from build123d import *

# Parameters (mm, degrees)
SKETCH_1_W          = 7
SKETCH_1_H          = 13
SKETCH_1_H_2        = 2
EXTRUDE_1_DEPTH     = 7
SKETCH_2_W          = 7
SKETCH_2_H          = 7
CUT_EXTRUDE_1_DEPTH = 3.5
FILLET_1_R          = 3.5
SKETCH_3_R          = 1.5
CUT_EXTRUDE_2_DEPTH = 13.835497653
SKETCH_4_R          = 1.5
CUT_EXTRUDE_3_DEPTH = 17.740669043
FILLET_2_R          = 2
FILLET_3_R          = 0.8


with BuildPart() as part:
    # 草图1 → 凸台-拉伸1 (new body)
    with BuildSketch(Plane.XY):
        with BuildLine():
            Line((-8.5, -6.5), (-3.5, -6.5))
            Line((-3.5, -6.5), (-3.5, -1.5))
            ThreePointArc((-3.5, -1.5), (-4.964466094, -5.035533906), (-8.5, -6.5))
        make_face()
        Rectangle(SKETCH_1_W, SKETCH_1_H)
        with Locations((7, -5.5)):
            Rectangle(SKETCH_1_W, SKETCH_1_H_2)
    extrude(amount=EXTRUDE_1_DEPTH)

    # 草图2 → 切除-拉伸1 (cut)
    with BuildSketch(Plane.XY.offset(7)):
        with Locations((0, 3)):
            Rectangle(SKETCH_2_W, SKETCH_2_H)
    extrude(amount=-CUT_EXTRUDE_1_DEPTH, mode=Mode.SUBTRACT)

    # 圆角1
    fillet_1_edges = [part.edges().sort_by_distance(p)[0] for p in [
        (10.5, -5.5, 0),
        (10.5, -5.5, 7),
        (3.5, 6.5, 1.75),
        (-3.5, 6.5, 1.75),
    ]]
    fillet(fillet_1_edges, radius=FILLET_1_R - 0.0001)  # a hair under: the kernel refuses the full size

    # 草图3 → 切除-拉伸2 (cut, through all)
    with BuildSketch(Plane.XY.offset(3.5)):
        with Locations((0, 3)):
            Circle(SKETCH_3_R)
    extrude(amount=-CUT_EXTRUDE_2_DEPTH, mode=Mode.SUBTRACT)

    # 草图4 → 切除-拉伸3 (cut, through all)
    with BuildSketch(Plane(origin=(0, -4.5, 0), x_dir=(1, 0, 0), z_dir=(0, 1, 0))):
        with Locations(Location((7, -3.5, 0), (0, 0, 180))):
            Circle(SKETCH_4_R)
    extrude(amount=-CUT_EXTRUDE_3_DEPTH, mode=Mode.SUBTRACT)

    # 圆角2
    fillet_2_edges = [part.edges().sort_by_distance(p)[0] for p in [
        (3.5, -4.5, 3.5),
    ]]
    fillet(fillet_2_edges, radius=FILLET_2_R - 0.0001)  # a hair under: the kernel refuses the full size

    # 圆角3
    fillet_3_edges = [part.edges().sort_by_distance(p)[0] for p in [
        (-4.964466094, -5.035533906, 0),
        (3.5, -1.50005, 7),
        (-3.5, -1, 7),
        (0, -0.5, 7),
        (-4.964466094, -5.035533906, 7),
        (6.25, -4.5, 0),
        (6.25, -4.5, 7),
        (9.474903023, -4.5, 5.974903023),
        (9.474903023, -4.5, 1.025096977),
        (-3.5, 0.75005, 0),
        (3.5, 0.25, 0),
        (-2.474903023, 5.474903023, 0),
        (2.474903023, 5.474903023, 0),
        (4.085757148, -3.914242852, 0),
        (4.085757148, -3.914242852, 7),
    ]]
    fillet(fillet_3_edges, radius=FILLET_3_R)


solid = part.part
Read the model definition and answer for the solid it produces. Units are mm, in the model's axes. A direction names the side the tool comes from. Round coordinates to 2 decimals unless told otherwise and drop trailing zeros. Write each loop counter-clockwise with the first axis right and the second up, starting at its lowest first coordinate (ties: lowest second). Pieces come first, ordered by that corner, then holes. Notation, with made-up numbers: M 22.25,43 L 34.25,43 A31 cw 34.25,77 Z; hole C 35.25,-13.5 d4. An arc over 180 degrees is marked long. Use a Markdown table: item, result.
1) For a pull along Z with two mould halves and no side action, classify faces 6 (the cylindrical face through (6.24, -4.74, 0.23)), 7 (the cylindrical face through (8.5, -5.49, 3.57)), 8 (the flat face through (-3.5, 0, 3)) as pulls with the +Z half, pulls with the -Z half, needs draft (parallel to the pull), parting line crosses it, or undercut.
Answers follow:
| item | result |
|---|---|
| face 6 | pulls with the -Z half |
| face 7 | undercut |
| face 8 | needs draft |
2) The part is cut by section B-B (x = 6). Write down the section's boundary in (y, z), plus the area to 3 significant figures.
Answers follow:
| item | result |
|---|---|
| outline | M -6.5,0 L -5.3,0 A0.8 ccw -4.5,0.8 L -4.5,2.38 L -6.5,2.38 Z; M -6.5,4.62 L -4.5,4.62 L -4.5,6.2 A0.8 ccw -5.3,7 L -6.5,7 Z |
| area | 9.25 mm2 |
3) Flat-ended cylindrical pins translate along their axes: pin 1 (2 mm diameter, centred on x = 0, z = 6, fed in from +Y); pin 2 (3.5 mm diameter, centred on x = 7.5, z = 2.5, fed in from +Y); pin 3 (2.5 mm diameter, centred on y = 0.5, z = 2.5, fed in from -X); pin 4 (1.8 mm diameter, centred on x = 7, z = 3.5, fed in from -Y). Find the tip coordinate at first contact, or state that the pin passes through.
Answers follow:
| item | result |
|---|---|
| pin 1 | stops at y = -0.5 |
| pin 2 | stops at y = -4.5 |
| pin 3 | stops at x = -3.5 |
| pin 4 | passes through |
4) The part is cut by section C-C (y = 1). Write down the section's boundary in (x, z), plus the area to 3 significant figures.
Answers follow:
| item | result |
|---|---|
| outline | M -3.5,0.8 A0.8 ccw -2.7,0 L 2.7,0 A0.8 ccw 3.5,0.8 L 3.5,3.5 L -3.5,3.5 Z |
| area | 24.2 mm2 |
5) Straight lines are drawn through the part: line 1 along Z through (x, y) = (7, -5.7); line 2 along Y through (x, z) = (0, 2.2); line 3 along Z through (x, y) = (2.25, 3.5). For each, find the intervals that lie inside material, in ascending order. Write a range as [from, to].
Answers follow:
| item | result |
|---|---|
| line 1 | z = [0, 2], [5, 7] |
| line 2 | y = [-6.5, 1.5], [4.5, 6.5] |
| line 3 | z = [0, 3.5] |
6) The part is cut by section A-A (y = 2.75). Write down the section's boundary in (x, z).
Answers follow:
| item | result |
|---|---|
| outline | M -3.5,0.8 A0.8 ccw -2.7,0 L -1.48,0 L -1.48,3.5 L -3.5,3.5 Z; M 1.48,0 L 2.7,0 A0.8 ccw 3.5,0.8 L 3.5,3.5 L 1.48,3.5 Z |
7) A tool of negligible diameter and unlimited length cuts with its end or side. For faces 1 (the flat face through (0, 1, 3.5)), 2 (the cylindrical face through (6.26, -4.74, 6.77)), 3 (the cylindrical face through (-3.36, -1.1, 6.65)), 4 (the cylindrical face through (9.5, -5.89, 5.95)), 5 (the flat face through (3.5, 0, 3)), from which of +Z, -Z, +X, -X, +Y, -Y can it reach the whole face along a straight path? Write none if from no direction.
Answers follow:
| item | result |
|---|---|
| face 1 | +Z, +X, -X, +Y |
| face 2 | +Z, +X, +Y |
| face 3 | +Z, -X, +Y |
| face 4 | +Z, +X, +Y, -Y |
| face 5 | +Z, -Z, +X, +Y |
